Input: part model. Units: mm. Frame: model coordinates. A direction names the side the tool comes from. Give positions to 0.01 mm unless a question says otherwise; leave off trailing zeros. Loops run counter-clockwise (first coordinate to the right, second up) from the corner with the lowest first, then second, coordinate; pieces in that order, holes last. Notation, with made-up numbers: (-40, -25) -> (10, -25) arc R14 ccw to (10, -15) -> close; hole circle Ø11 at (63, -29). An arc over 180 degrees is marked (long way). Answer as a JSON object with one key per item and string values.
```python
from build123d import *

# Parameters (mm, degrees)
F0_R     = 31.75
F0_W     = 40.64
F0_H     = 30.48
F1_DEPTH = 2.54
F2_DEPTH = 15.24


with BuildPart() as f1:
    # F0 (on Front) → F1 (new body)
    with BuildSketch(Plane.XZ):
        Circle(F0_R)
        with Locations((0.068977, 0)):
            Rectangle(F0_W, F0_H, mode=Mode.SUBTRACT)
    extrude(amount=F1_DEPTH)

    # F0 (on Front) → F2 (join)
    with BuildSketch(Plane.XZ):
        with Locations((0.068977, 0)):
            Rectangle(F0_W, F0_H)
    extrude(amount=F2_DEPTH)


solid = f1.part
```
Q1. Ray query, line 1 along Z through (x, y) = (14, -7.75); line 2 along X through (y, z) = (-10, 14); line 3 along Y through (x, z) = (6.5, 18.5). Return the intervals inside material, ascending.
Evaluation:
{"line 1": "z = -15.24 to 15.24", "line 2": "x = -20.25 to 20.39", "line 3": "y = -2.54 to 0"}
Q2. Section A-A, the plane z = 0. Return the cut outline in (x, y).
Evaluation:
{"outline": "(-31.75, -2.54) -> (-20.25, -2.54) -> (-20.25, -15.24) -> (20.39, -15.24) -> (20.39, -2.54) -> (31.75, -2.54) -> (31.75, 0) -> (-31.75, 0) -> close"}
Q3. Section B-B, the plane x = -15.5. Return the cut outline in (y, z), then the cut area to 3 significant figures.
Evaluation:
{"outline": "(-15.24, -15.24) -> (-2.54, -15.24) -> (-2.54, -27.71) -> (0, -27.71) -> (0, 27.71) -> (-2.54, 27.71) -> (-2.54, 15.24) -> (-15.24, 15.24) -> close", "area": "528 mm2"}
Q4. Access query for faces 1 (the flat face through (0, -9, -15.24)), 2 (the flat face through (-20.251, -9, 0)), 3 (the flat face through (20.389, -9, 0)), 4 (the flat face through (0, -15.24, 0)), 5 (the flat face through (0, -9, 15.24)). Directions: +Z, -Z, +X, -X, +Y, -Y. A direction counts if a zero-diameter tool reaches every point of the face in a straight line with its end or side. Return the directions, or none.
Evaluation:
{"face 1": "-Z, +X, -X, -Y", "face 2": "+Z, -Z, -X, -Y", "face 3": "+Z, -Z, +X, -Y", "face 4": "+Z, -Z, +X, -X, -Y", "face 5": "+Z, +X, -X, -Y"}
Q5. Section D-D, the plane x = -24.5. Return the cut outline in (y, z).
Evaluation:
{"outline": "(-2.54, -20.19) -> (0, -20.19) -> (0, 20.19) -> (-2.54, 20.19) -> close"}
Q6. Section C-C, the plane y = -12.5. Return the cut outline in (x, z), then the cut area to 3 significant figures.
Evaluation:
{"outline": "(-20.25, -15.24) -> (20.39, -15.24) -> (20.39, 15.24) -> (-20.25, 15.24) -> close", "area": "1,240 mm2"}
Q7. Pin query (flat end, axial travel): pin 1 (8 mm diameter, centred on x = 20.5, y = -2, fed in from -Z); pin 2 (3 mm diameter, centred on y = -9, z = -11, fed in from -X); pin 3 (1.5 mm diameter, centred on x = 3, y = -4.5, fed in from +Z). Return the tip coordinate at first contact, or that it passes through.
Evaluation:
{"pin 1": "stops at z = -27.13", "pin 2": "stops at x = -20.25", "pin 3": "stops at z = 15.24"}
